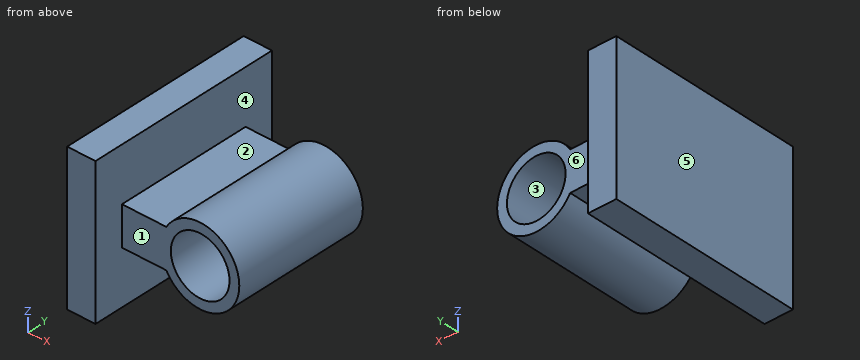
```python
from build123d import *

# Parameters (mm, degrees)
SKETCH1_W                = 15
SKETCH1_H                = 20
BOSS_EXTRUDE1_DEPTH      = 2.9
SKETCH2_W                = 1
SKETCH2_H                = 14
BOSS_EXTRUDE2_REACH      = 29.731
BOSS_EXTRUDE2_END_RADIUS = 4
SKETCH4_W                = 4
SKETCH4_H                = 14


with BuildPart() as part:
    # Sketch1 → Boss-Extrude1 (new body)
    with BuildSketch(Plane(origin=(0, 0, 0), x_dir=(0, 0, -1), z_dir=(1, 0, 0))):
        with Locations((7.5, 10)):
            Rectangle(SKETCH1_W, SKETCH1_H)
    extrude(amount=BOSS_EXTRUDE1_DEPTH)



with BuildPart() as body_2:
    # Sketch2 → Revolve1 (revolve)
    with BuildSketch(Plane(origin=(10.9, 0, 0), x_dir=(0, 0, -1), z_dir=(1, 0, 0))):
        with Locations((11, 10)):
            Rectangle(SKETCH2_W, SKETCH2_H)
    revolve(axis=Axis((10.9, 0, -7.5), (0, 1, 0)))


with BuildPart() as part_1:
    add(part.part)

    add(body_2.part)  # Boss-Extrude2 merges body 2
    # Boss-Extrude2: up to this cylinder (the profile starts outside it)
    boss_extrude2_end = Plane(origin=(10.9, 10, -7.5), z_dir=(0, -1, 0)) * Cylinder(BOSS_EXTRUDE2_END_RADIUS, 68.462, mode=Mode.PRIVATE)
    # Sketch4 → Boss-Extrude2 (add, up to the surface)
    with BuildSketch(Plane(origin=(2.9, 0, 0), x_dir=(0, 0, -1), z_dir=(1, 0, 0)), mode=Mode.PRIVATE) as boss_extrude2_sk1:
        with Locations((7.5, 10)):
            Rectangle(SKETCH4_W, SKETCH4_H)
    boss_extrude2_tool1 = extrude(boss_extrude2_sk1.sketch, amount=BOSS_EXTRUDE2_REACH, mode=Mode.PRIVATE) - boss_extrude2_end
    add(boss_extrude2_tool1.solids().sort_by_distance((2.9, 10, -7.5))[0])


solid = part_1.part
```
Could you check a few things on this model? Use its own coordinates, in mm. Face numbers are marked on the shaded views. A direction names the side the tool comes from. Coordinates: 2 decimals unless noted, no trailing zeros. Loops run counter-clockwise (first coordinate to the right, second up) from the corner with the lowest first, then second, coordinate; pieces in that order, holes last. Notation, with made-up numbers: M 68.5,-19 L 100.5,-19 A35 cw 100.5,14 Z; hole C -12,12 d6. An arc over 180 degrees is marked long. Put each result on its own line as item: value. Start each with the question number.
(1) Thinking about a two-plate mould opening in X: for the marked faces 4, 5 and 6, which applies, pulls with the +X half, pulls with the -X half, needs draft (parallel to the pull), parting line crosses it, or undercut?
(2) For the marked faces 1, 2 and 3, which set-ups out of +Z, -Z, +X, -X, +Y, -Y let a thin tool reach every point of the face, with its end or its side?
(3) Suppose I cut it at D-D on z = -4.75. Please give me the cut outline in (x, y), then the cut area to 3 significant figures.
(4) Suppose I cut it at B-B on x = 10.9. Please give me the cut outline in (y, z).
(5) Suppose I cut it at C-C on y = 3.75. Please give me the cut outline in (x, z), then the cut area to 3 significant figures.
(6) Suppose I cut it at A-A on z = -7.5. Please give me the cut outline in (x, y).
(7) Will these pins go through, and if not, where does the flat tip stop? P1, Ø5.5, axis at x = 10.9, z = -7.5, coming from the -Y side; P2, Ø1.4, axis at x = 5, y = 6.5, coming from the +Z side; P3, Ø4, axis at x = 7, z = -5.5, coming from the +Y side; P4, Ø3, axis at y = 18, z = -7.5, coming from the +X side.
(8) I need wall thicknesses on line 1 (Z direction, x = 10.9, y = 6.5); line 2 (X direction, y = 11, z = -5); line 3 (X direction, y = 14.25, z = -7.5). Which ranges of each line are inside material? Lowest first, please. Write a range as from..to.
Solutions:
1. face 4: undercut
1. face 5: pulls with the -X half
1. face 6: needs draft
2. face 1: +Z, -Z, +X, -Y
2. face 2: +Z, +Y, -Y
2. face 3: +Y, -Y
3. outline: M 0,0 L 2.9,0 L 2.9,20 L 0,20 Z; M 8,3 L 9.7,3 L 9.7,17 L 8,17 Z; M 12.1,3 L 13.8,3 L 13.8,17 L 12.1,17 Z
3. area: 106 mm2
4. outline: M 3,-11.5 L 17,-11.5 L 17,-10.5 L 3,-10.5 Z; M 3,-4.5 L 17,-4.5 L 17,-3.5 L 3,-3.5 Z
5. outline: M 0,-15 L 2.9,-15 L 2.9,-9.5 L 7.44,-9.5 A4 ccw long 7.44,-5.5 L 2.9,-5.5 L 2.9,0 L 0,0 Z; hole C 10.9,-7.5 d6
5. area: 82.2 mm2
6. outline: M 0,0 L 2.9,0 L 2.9,3 L 7.9,3 L 7.9,17 L 2.9,17 L 2.9,20 L 0,20 Z; M 13.9,3 L 14.9,3 L 14.9,17 L 13.9,17 Z
7. P1: passes through
7. P2: stops at z = -5.5
7. P3: stops at y = 17
7. P4: stops at x = 14.9
8. line 1: z = -11.5..-10.5, -4.5..-3.5
8. line 2: x = 0..2.9, 7.78..9.24, 12.56..14.02
8. line 3: x = 0..7.9, 13.9..14.9
